```python
from build123d import *

# Parameters (mm, degrees)
F0_R          = 3
F0_R_2        = 2.5
F1_DEPTH      = 250
F2_R          = 2
F3_R          = 7
F5_DEPTH      = 30
F5_DEPTH_BACK = 30


# Not quite as in the source:
# - a feature names something its author has since deleted; it is built from what else it names


with BuildPart() as f1:
    # F0 (on Top) → F1 (new body)
    with BuildSketch(Plane.XY):
        with BuildLine():
            Line((18.15, -30), (30, -30))
            Line((30, -30), (30, -18.15))
            Line((30, -18.15), (27.5, -18.15))
            Line((27.5, -18.15), (27.5, -20.15))
            Line((27.5, -20.15), (21.5477069044, -20.15))
            ThreePointArc((21.5477069044, -20.15), (19.5, -15), (21.5477069044, -9.85))
            Line((21.5477069044, -9.85), (27.5, -9.85))
            Line((27.5, -9.85), (27.5, -11.85))
            Line((27.5, -11.85), (30, -11.85))
            Line((30, -11.85), (30, 11.85))
            Line((30, 11.85), (27.5, 11.85))
            Line((27.5, 11.85), (27.5, 9.85))
            Line((27.5, 9.85), (21.5477069044, 9.85))
            ThreePointArc((21.5477069044, 9.85), (19.5, 15), (21.5477069044, 20.15))
            Line((21.5477069044, 20.15), (27.5, 20.15))
            Line((27.5, 20.15), (27.5, 18.15))
            Line((27.5, 18.15), (30, 18.15))
            Line((30, 18.15), (30, 30))
            Line((30, 30), (18.15, 30))
            Line((18.15, 30), (18.15, 27.5))
            Line((18.15, 27.5), (20.15, 27.5))
            Line((20.15, 27.5), (20.15, 21.5477069044))
            ThreePointArc((20.15, 21.5477069044), (15, 19.5), (9.85, 21.5477069044))
            Line((9.85, 21.5477069044), (9.85, 27.5))
            Line((9.85, 27.5), (11.85, 27.5))
            Line((11.85, 27.5), (11.85, 30))
            Line((11.85, 30), (-11.85, 30))
            Line((-11.85, 30), (-11.85, 27.5))
            Line((-11.85, 27.5), (-9.85, 27.5))
            Line((-9.85, 27.5), (-9.85, 21.5477069044))
            ThreePointArc((-9.85, 21.5477069044), (-15, 19.5), (-20.15, 21.5477069044))
            Line((-20.15, 21.5477069044), (-20.15, 27.5))
            Line((-20.15, 27.5), (-18.15, 27.5))
            Line((-18.15, 27.5), (-18.15, 30))
            Line((-18.15, 30), (-30, 30))
            Line((-30, 30), (-30, 18.15))
            Line((-30, 18.15), (-27.5, 18.15))
            Line((-27.5, 18.15), (-27.5, 20.15))
            Line((-27.5, 20.15), (-21.5477069044, 20.15))
            ThreePointArc((-21.5477069044, 20.15), (-19.5, 15), (-21.5477069044, 9.85))
            Line((-21.5477069044, 9.85), (-27.5, 9.85))
            Line((-27.5, 9.85), (-27.5, 11.85))
            Line((-27.5, 11.85), (-30, 11.85))
            Line((-30, 11.85), (-30, -11.85))
            Line((-30, -11.85), (-27.5, -11.85))
            Line((-27.5, -11.85), (-27.5, -9.85))
            Line((-27.5, -9.85), (-21.5477069044, -9.85))
            ThreePointArc((-21.5477069044, -9.85), (-19.5, -15), (-21.5477069044, -20.15))
            Line((-21.5477069044, -20.15), (-27.5, -20.15))
            Line((-27.5, -20.15), (-27.5, -18.15))
            Line((-27.5, -18.15), (-30, -18.15))
            Line((-30, -18.15), (-30, -30))
            Line((-30, -30), (-18.15, -30))
            Line((-18.15, -30), (-18.15, -27.5))
            Line((-18.15, -27.5), (-20.15, -27.5))
            Line((-20.15, -27.5), (-20.15, -21.5477069044))
            ThreePointArc((-20.15, -21.5477069044), (-15, -19.5), (-9.85, -21.5477069044))
            Line((-9.85, -21.5477069044), (-9.85, -27.5))
            Line((-9.85, -27.5), (-11.85, -27.5))
            Line((-11.85, -27.5), (-11.85, -30))
            Line((-11.85, -30), (11.85, -30))
            Line((11.85, -30), (11.85, -27.5))
            Line((11.85, -27.5), (9.85, -27.5))
            Line((9.85, -27.5), (9.85, -21.5477069044))
            ThreePointArc((9.85, -21.5477069044), (15, -19.5), (20.15, -21.5477069044))
            Line((20.15, -21.5477069044), (20.15, -27.5))
            Line((20.15, -27.5), (18.15, -27.5))
            Line((18.15, -27.5), (18.15, -30))
        make_face()
        with Locations((-25, -25)):
            Circle(F0_R, mode=Mode.SUBTRACT)
        with Locations((-15, -15)):
            Circle(F0_R_2, mode=Mode.SUBTRACT)
        with Locations((25, -25)):
            Circle(F0_R, mode=Mode.SUBTRACT)
        with Locations((15, -15)):
            Circle(F0_R_2, mode=Mode.SUBTRACT)
        with Locations((-25, 25)):
            Circle(F0_R, mode=Mode.SUBTRACT)
        with Locations((-15, 15)):
            Circle(F0_R_2, mode=Mode.SUBTRACT)
        Polygon((-7, 22), (-7, 27.5), (0, 27.5), (7, 27.5), (7, 22), (10, 16), (10, 10), (16, 10), (22, 7), (27.5, 7), (27.5, 0), (27.5, -7), (22, -7), (16, -10), (10, -10), (10, -16), (7, -22), (7, -27.5), (0, -27.5), (-7, -27.5), (-7, -22), (-10, -16), (-10, -10), (-16, -10), (-22, -7), (-27.5, -7), (-27.5, 0), (-27.5, 7), (-22, 7), (-16, 10), (-10, 10), (-10, 16), align=None, mode=Mode.SUBTRACT)
        with Locations((15, 15)):
            Circle(F0_R_2, mode=Mode.SUBTRACT)
        with Locations((25, 25)):
            Circle(F0_R, mode=Mode.SUBTRACT)
    extrude(amount=F1_DEPTH)

    # F2
    f2_edges = [f1.edges().sort_by_distance(p)[0] for p in [
        (-7, 27.5, 125),
        (7, 27.5, 125),
    ]]
    fillet(f2_edges, radius=F2_R)

    # F3
    f3_edges = [f1.edges().sort_by_distance(p)[0] for p in [
        (-10, 16, 125),
        (10, 16, 125),
    ]]
    fillet(f3_edges, radius=F3_R)

    # F4 (on Right) → F5 (cut, two sides)
    with BuildSketch(Plane.YZ) as f5_sk:
        Polygon((-23.2563562234, -128.5722174771), (30, 0), (-168.5306378236, 82.2340827331), (-221.786994047, -46.338134744), align=None)
        Polygon((171.7491592878, 324.7994275924), (-8.0091289948, 360.5555742708), (-30, 250), (149.7582882826, 214.2438533216), align=None)
    extrude(amount=F5_DEPTH, mode=Mode.SUBTRACT)
    extrude(f5_sk.sketch, amount=-F5_DEPTH_BACK, mode=Mode.SUBTRACT)


solid = f1.part
```
Can you work these out from the model? Positions are in its coordinate system, mm. Coordinates: 2 decimals unless noted, no trailing zeros. Order: outer loops, then holes, each group sorted by start corner. A loop starts at its lowest first (then second) coordinate and runs counter-clockwise, first axis right, second up.
1. I'm going to push a flat-ended pin straight in: pin 1 (3 mm diameter, centred on x = -10.5, y = -13, fed in from -Z). Where does the tip first touch, or does it pass through?
2. If we section it at B-B (y = 1): Please give me the cut outline in (x, z), then the cut area to 3 significant figures.
3. I need wall thicknesses on line 1 (X direction, y = 25, z = 135); line 2 (X direction, y = 15, z = 94.5); line 3 (Y direction, x = -15, z = 105.5). Which ranges of each line are inside material? Lowest first, please.
4. If we section it at D-D (x = 24.5): Please give me the cut outline in (y, z), then the cut area to 3 significant figures.
5. If we section it at A-A (x = -1): Please give me the cut outline in (y, z), then the cut area to 3 significant figures.
6. If we section it at C-C (y = -25): Please give me the cut outline in (x, z).
7. Thinking about a two-plate mould opening in Y: for faces 1 (the face through (-19, 8.5, 123.8)), 2 (the face through (-30, 24, 119)), which applies, +Y half, -Y half, draft (parallel to the pull), parting line (faces both ways), or undercut?
Entries:
1. pin 1: stops at z = 17.19
2. outline: (-30, 12.01) - (-27.5, 12.01) - (-27.5, 243.83) - (-30, 243.83) - close; (27.5, 12.01) - (30, 12.01) - (30, 243.83) - (27.5, 243.83) - close
2. area: 1,160 mm2
3. line 1: x = -30 to -28, -22 to -20.15, -9.85 to -7, 7 to 9.85, 20.15 to 22, 28 to 30
3. line 2: x = -19.5 to -17.5, -12.5 to -9.97, 9.97 to 12.5, 17.5 to 19.5
3. line 3: y = -19.5 to -17.5, -12.5 to -10, 10 to 12.5, 17.5 to 19.5
4. outline: (-30, 24.85) - (-27.96, 24.01) - (-27.96, 249.59) - (-30, 250) - close; (-22.04, 21.56) - (-20.15, 20.77) - (-20.15, 248.04) - (-22.04, 248.42) - close; (-9.85, 16.51) - (-7, 15.33) - (-7, 245.43) - (-9.85, 245.99) - close; (7, 9.53) - (9.85, 8.35) - (9.85, 242.07) - (7, 242.64) - close; (20.15, 4.08) - (22.04, 3.3) - (22.04, 239.65) - (20.15, 240.02) - close; (27.96, 0.85) - (30, 0) - (30, 238.07) - (27.96, 238.47) - close
4. area: 3,140 mm2
5. outline: (-30, 24.85) - (-27.5, 23.82) - (-27.5, 249.5) - (-30, 250) - close; (27.5, 1.04) - (30, 0) - (30, 238.07) - (27.5, 238.56) - close
5. area: 1,160 mm2
6. outline: (-30, 22.78) - (-28, 22.78) - (-28, 249.01) - (-30, 249.01) - close; (-22, 22.78) - (-20.15, 22.78) - (-20.15, 249.01) - (-22, 249.01) - close; (-9.85, 22.78) - (-7, 22.78) - (-7, 249.01) - (-9.85, 249.01) - close; (7, 22.78) - (9.85, 22.78) - (9.85, 249.01) - (7, 249.01) - close; (20.15, 22.78) - (22, 22.78) - (22, 249.01) - (20.15, 249.01) - close; (28, 22.78) - (30, 22.78) - (30, 249.01) - (28, 249.01) - close
7. face 1: undercut
7. face 2: draft
